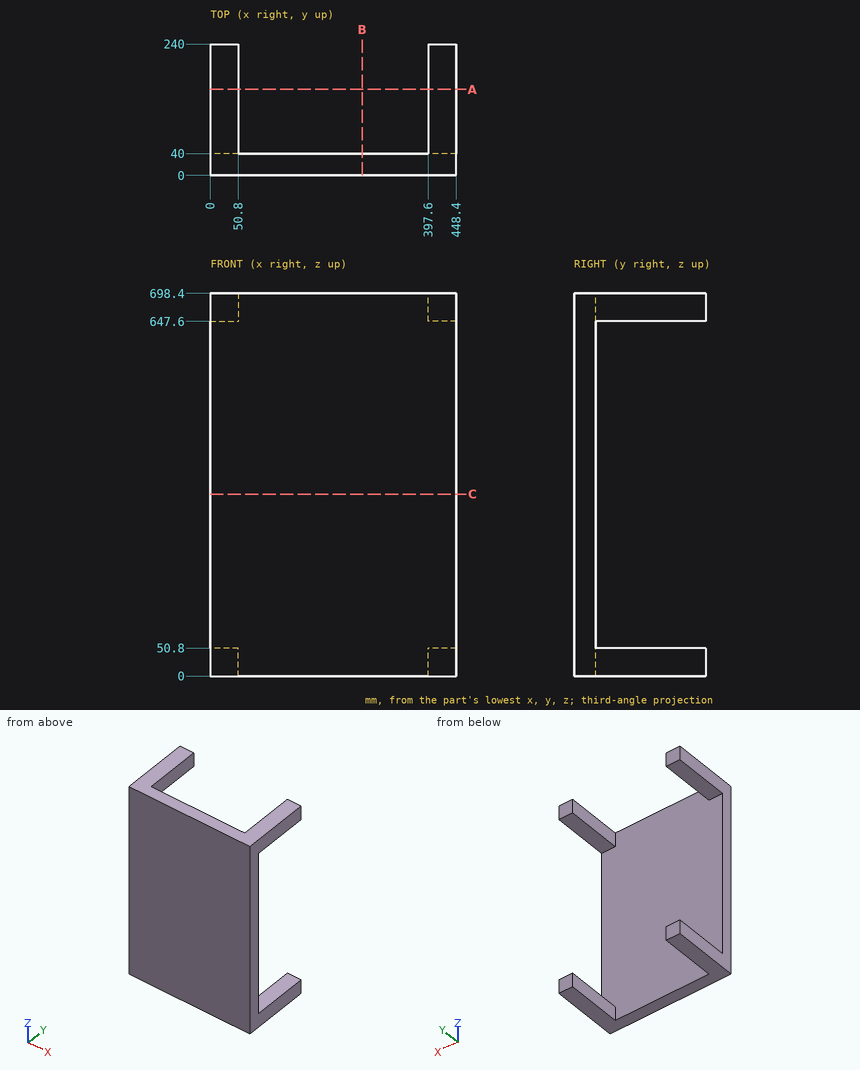
Design review of the part shown in the three views and the two pictorial views. Dimensions are in mm from the part's minimum x, y and z. Round coordinates to 2 decimals unless told otherwise and drop trailing zeros. Loops run counter-clockwise (first coordinate to the right, second up) from the corner with the lowest first, then second, coordinate; pieces in that order, holes last. Notation, with made-up numbers: M 39.5,-34.75 L 64.5,-34.75 A26 ccw 64.5,-14.75 Z; hole C -21.75,-5 d3. An arc over 180 degrees is marked long. Answer as a JSON object with one key per item and string values.
Item 1: We need section B-B, the plane x = 277. State the section outline as (y, z) points, and give its area (3 significant figures).
Check sheet entries:
{"outline": "M 0,0 L 40,0 L 40,698.4 L 0,698.4 Z", "area": "27,900 mm2"}
Item 2: For line 1 along Z through (x, y) = (30, 199); line 2 along X through (y, z) = (151, 669.5); line 3 along Y through (x, z) = (163, 139), list the stretches that pass through material, from the lowest coordinate up.
Check sheet entries:
{"line 1": "0 to 50.8, 647.6 to 698.4", "line 2": "0 to 50.8, 397.6 to 448.4", "line 3": "0 to 40"}
Item 3: We need section A-A, the plane y = 157. State the section outline as (x, z) points.
Check sheet entries:
{"outline": "M 0,0 L 50.8,0 L 50.8,50.8 L 0,50.8 Z; M 0,647.6 L 50.8,647.6 L 50.8,698.4 L 0,698.4 Z; M 397.6,0 L 448.4,0 L 448.4,50.8 L 397.6,50.8 Z; M 397.6,647.6 L 448.4,647.6 L 448.4,698.4 L 397.6,698.4 Z"}
Item 4: Clearance check with flat-ended pins moving along their axes: P1, Ø15, axis at x = 434.5, y = 156.5, coming from the -Z side; P2, Ø8, axis at x = 334, z = 485, coming from the +Y side. State where each tip first meets the part, or that it passes through.
Check sheet entries:
{"P1": "z = 0", "P2": "y = 40"}
Item 5: We need section C-C, the plane z = 332. State the section outline as (x, y) points.
Check sheet entries:
{"outline": "M 0,0 L 448.4,0 L 448.4,40 L 0,40 Z"}
